For this review, take the finished solid that the model builds, in its own axes (mm). A direction names the side the tool comes from. Coordinates: 2 decimals unless noted, no trailing zeros. Loops run counter-clockwise (first coordinate to the right, second up) from the corner with the lowest first, then second, coordinate; pieces in that order, holes last.
```python
from build123d import *

# Parameters (mm, degrees)
SZKIC1_W                                             = 320
SZKIC1_H                                             = 420
DODANIE_WYCI_GNI_CIE1_DEPTH                          = 14
POG_BIENIE_WALCOWE_POD_M5_WKR_T_DO_CZ_CI_D           = 5.5
POG_BIENIE_WALCOWE_POD_M5_WKR_T_DO_CZ_CI_CBORE_D     = 9
POG_BIENIE_WALCOWE_POD_M5_WKR_T_DO_CZ_CI_CBORE_DEPTH = 6
SZKIC10_W                                            = 70
SZKIC10_H                                            = 4
WYTNIJ_WYCI_GNI_CIE1_DEPTH                           = 50
ZAOKR_GLENIE1_R                                      = 10
SKETCH_1_R                                           = 4.5
CUT_EXTRUDE_1_DEPTH                                  = 6
SKETCH_2_R                                           = 2.75
CUT_EXTRUDE_2_DEPTH                                  = 265.378516525


with BuildPart() as part:
    # Szkic1 → Dodanie-wyciągnięcie1 (new body)
    with BuildSketch(Plane(origin=(0, 0, 0), x_dir=(1, 0, 0), z_dir=(0, 1, 0))):
        Rectangle(SZKIC1_W, SZKIC1_H)
    extrude(amount=DODANIE_WYCI_GNI_CIE1_DEPTH)

    # Pogłębienie walcowe pod M5 Wkręt do części metalowych z łbem sześciokątnym1 (through all)
    with Locations(Plane(origin=(0, 14, 0), x_dir=(1, 0, 0), z_dir=(0, 1, 0))):
        with Locations((-87.5, -141), (-87.5, -109), (-57.5, -141), (-57.5, -109), (57.5, -141), (57.5, -109), (87.5, -109), (87.5, -141)):
            pog_bienie_walcowe_pod_m5_wkr_t_do_cz_ci = CounterBoreHole(POG_BIENIE_WALCOWE_POD_M5_WKR_T_DO_CZ_CI_D / 2, POG_BIENIE_WALCOWE_POD_M5_WKR_T_DO_CZ_CI_CBORE_D / 2, POG_BIENIE_WALCOWE_POD_M5_WKR_T_DO_CZ_CI_CBORE_DEPTH)

    # Lustro3: Pogłębienie walcowe pod M5 Wkręt do części metalowych z łbem sześciokątnym1 across plane
    add(pog_bienie_walcowe_pod_m5_wkr_t_do_cz_ci.mirror(Plane.XY), mode=Mode.SUBTRACT)

    # Szkic10 → Wytnij-wyciągnięcie1 (cut)
    with BuildSketch(Plane.ZY.offset(160)):
        with Locations((0, 2)):
            Rectangle(SZKIC10_W, SZKIC10_H)
    extrude(amount=-WYTNIJ_WYCI_GNI_CIE1_DEPTH, mode=Mode.SUBTRACT)

    # Zaokrąglenie1
    zaokr_glenie1_edges = [part.edges().sort_by_distance(p)[0] for p in [
        (-110, 2, -35),
        (-110, 2, 35),
    ]]
    fillet(zaokr_glenie1_edges, radius=ZAOKR_GLENIE1_R)

    # 草图1 → 切除-拉伸1 (cut)
    with BuildSketch(Plane(origin=(0, 14, 0), x_dir=(1, 0, 0), z_dir=(0, 1, 0))):
        with Locations(Location((11.5, 32, 0), (0, 0, 270))):
            Circle(SKETCH_1_R)
        with Locations(Location((-11.5, 32, 0), (0, 0, 90))):
            Circle(SKETCH_1_R)
        with Locations(Location((-11.5, -32, 0), (0, 0, 270))):
            Circle(SKETCH_1_R)
        with Locations(Location((11.5, -32, 0), (0, 0, 90))):
            Circle(SKETCH_1_R)
    extrude(amount=-CUT_EXTRUDE_1_DEPTH, mode=Mode.SUBTRACT)

    # 草图2 → 切除-拉伸2 (cut, through all)
    with BuildSketch(Plane(origin=(0, 14, 0), x_dir=(1, 0, 0), z_dir=(0, 1, 0))):
        with Locations(Location((11.5, 32, 0), (0, 0, 270))):
            Circle(SKETCH_2_R)
        with Locations(Location((-11.5, 32, 0), (0, 0, 90))):
            Circle(SKETCH_2_R)
        with Locations(Location((-11.5, -32, 0), (0, 0, 270))):
            Circle(SKETCH_2_R)
        with Locations(Location((11.5, -32, 0), (0, 0, 90))):
            Circle(SKETCH_2_R)
    extrude(amount=-CUT_EXTRUDE_2_DEPTH, mode=Mode.SUBTRACT)


solid = part.part
```
Q1. Consider section B-B (z = 17.5). State the section outline as (x, y) points, then the cut area to 3 significant figures.
Q2. Machinability: for faces 1 (the face through (-135, 4, 0)), 2 (the face through (-90, 8, 143)), which of the approach directions +Z, -Z, +X, -X, +Y, -Y give a long, thin tool a straight path to every point of the face, cutting with its end or side? Answer none if there is none.
Q3. Wall thickness on probe 1 along Z at (x, y) = (57.5, 3.5); probe 2 along X at (y, z) = (3, -109); probe 3 along X at (y, z) = (12.1, 141): over which ranges is each line inside the solid? List them lowest first.
Q4. Consider section A-A (x = -115). State the section outline as (y, z) points, then the cut area to 3 significant figures.
Q5. The part is to be moulded in two halves that separate along Z. For faces 3 (the face through (-160, 7, 3)), 4 (the face through (10.148, 11.042, 27.708)), 5 (the face through (84.18, 11.04, -105.96)), say which applies: +Z half, -Z half, draft (parallel to the pull), parting line (faces both ways), or undercut.
Q6. For pin 1 Ø6.5 at (x, z) = (-57.5, -109) entering from +Y; pin 2 Ø14.5 at (x, z) = (-87.5, 109) entering from -Y; pin 3 Ø5 at (x, z) = (87.5, -109) entering from -Y, all flat-tipped, find the tip position at first contact; note any pin that passes through.
Model answer:
1. outline: (-160, 4) - (-110, 4) - (-110, 0) - (160, 0) - (160, 14) - (-160, 14) - close
1. area: 4,280 mm2
2. face 1: -X, -Y
2. face 2: +Y
3. probe 1: z = -210 to -143.75, -138.25 to -111.75, -106.25 to 106.25, 111.75 to 138.25, 143.75 to 210
3. probe 2: x = -160 to -90.25, -84.75 to -60.25, -54.75 to 54.75, 60.25 to 84.75, 90.25 to 160
3. probe 3: x = -160 to -92, -83 to -62, -53 to 53, 62 to 83, 92 to 160
4. outline: (0, -210) - (14, -210) - (14, 210) - (0, 210) - (0, 33.66) - (4, 33.66) - (4, -33.66) - (0, -33.66) - close
4. area: 5,610 mm2
5. face 3: draft
5. face 4: undercut
5. face 5: undercut
6. pin 1: stops at y = 8
6. pin 2: stops at y = 0
6. pin 3: passes through
